Autodesk Inventor part; units mm, degrees
sketch "Эскиз1" plane through (0, 0, 0) normal (1, 0, 0) x (0, 1, 0)
  line L0 (-84.2261, 0) -> (14.4739, 0) construction
  circle A0 centre (-14.6261, 11.6003) radius 15
  line L1 (-70.1261, -37.7219) -> (-70.1261, 22.2781)
  line L2 (-70.1261, -37.7219) -> (-9.6116, -2.5367)
  line L3 (-15.295, 26.5854) -> (-70.1261, 22.2781)
  line L4 (-70.1261, 36.1012) -> (-70.1261, -83.8988)
  line L5 (-70.1261, -37.7219) -> (-60.535, -54.2175)
  line L6 (-15.295, 26.5854) -> (-16.485, 41.7343)
  circle A1 centre (-10.3011, 0.4068) radius 1.05
  circle A2 centre (-19.4828, 0.6271) radius 1.05
  circle A3 centre (-25.8196, 7.2753) radius 1.05
  circle A4 centre (-25.5993, 16.4571) radius 1.05
  circle A5 centre (-18.9511, 22.7938) radius 1.05
  circle A6 centre (-9.7693, 22.5736) radius 1.05
  circle A7 centre (-3.4326, 15.9253) radius 1.05
  circle A8 centre (-3.6528, 6.7436) radius 1.05
  circle A9 centre (-14.6261, 11.6003) radius 6.1
  dimension "d21" = 60
  dimension "d24" = 70
  dimension "d25" = 55
  dimension "d26" = 59.825
  dimension "d29" = 12.2
extrude "Выдавливание3" add sketch "Эскиз1" along normal mid plane 50 contours A0 L3 | L2 L1 L3 A0 picked at (-14.2037, 20.8402)
sketch "Эскиз3" plane through (-25, -70.1261, -37.7219) normal (0, -1, 0) x (1, 0, 0)
  point P0 (25, 37.7219)
properties part number "Ушко петли крышки"
Build history of the part. All positions in model axes, mm. Coordinates: 2 decimals unless noted, no trailing zeros. Order: outer loops, then holes, each group sorted by start corner. A loop starts at its lowest first (then second) coordinate and runs counter-clockwise, first axis right, second up. Notation, with made-up numbers: M 29.5,14.5 L 44.5,14.5 A14 ccw 44.5,37.5 Z; hole C 46,0 d6. An arc over 180 degrees is marked long. One line per question, with ' | ' between items. Start each with the question number.
Q1. Two-plate mould, pull along Z, no slides. Class faces 1 (the face through (0, -70.126, -8)), 2 (the face through (-0.35, -2.95, 16.86)), 3 (the face through (-0.35, 0.036, 14.766)): +Z half, -Z half, draft (parallel to the pull), parting line (faces both ways), or undercut.
Q2. Saw through at B-B (x = -11). Count the separate pieces of the cut face and the enclosed holes in it, then the cut area to 3 significant figures.
Q3. Saw through at D-D (z = -13.5). List the corners of the cut face in (x, y).
Q4. Saw through at C-C (y = -33). List the corners of the cut face in (x, z).
Q5. Probe L1, parallel to Z at x = 23, y = -18; L2, parallel to Y at x = 21, z = -23; L3, parallel to Y at x = 0, z = 8.5. List the from-to ranges inside material, lowest first. Write a range as from..to.
Q6. Flat gauge pins, fed straight in: pin 1 Ø1.7 at (y, z) = (-25.6, 16.46) entering from +X; pin 2 Ø1 at (x, y) = (-12.5, -29) entering from -Z; pin 3 Ø8 at (x, y) = (8.5, -32.5) entering from -Z; pin 4 Ø1 at (x, z) = (-3.5, 7) entering from +Y. Where does each tip first touch, or does it go through?
Q7. Saw through at A-A (z = 10). List the corners of the cut face in (x, y), then the cut area to 3 significant figures.
Check values:
1) face 1: draft | face 2: undercut | face 3: parting line
2) separate pieces: 1 | enclosed holes: 9 | area: 2,770 mm2
3) outline: M -25,-70.13 L 25,-70.13 L 25,-28.47 L -25,-28.47 Z
4) outline: M -25,-16.14 L 25,-16.14 L 25,25.19 L -25,25.19 Z
5) L1: z = -7.41..6.52, 16.68..22.35, 23.24..26.37 | L2: y = -70.13..-44.81 | L3: y = -70.13..-19.88, -9.37..0.05
6) pin 1: passes through | pin 2: stops at z = -14.1 | pin 3: stops at z = -18.17 | pin 4: stops at y = -0.2
7) outline: M -25,-70.13 L 25,-70.13 L 25,-20.51 L -25,-20.51 Z; M -25,-8.74 L 25,-8.74 L 25,0.29 L -25,0.29 Z | area: 2,930 mm2
